Study the drawing (mm; zero at the part's minimum x, y, z) and answer. Coordinates: 2 decimals unless noted, no trailing zeros. Loops run counter-clockwise (first coordinate to the right, second up) from the corner with the lowest first, then second, coordinate; pieces in that order, holes last.
Q1. Straight lines are drawn through the part: line 1 (X direction, y = 62.5, z = 31) (1 decimal); line 2 (Y direction, x = 68, z = 68) (1 decimal); line 3 (Y direction, x = 60, z = 64) (1 decimal). For each, find the intervals that lie inside material, in ascending order.
Q2. Section A-A (z = 42) is taken. Give the vertices of the cut face in (x, y) (1 decimal).
Q3. The mould has two halves that part along X. Classify the marked faces 1 and 2: pulls with the +X half, pulls with the -X half, needs draft (parallel to the pull), parting line crosses it, or undercut.
Q4. Flat-ended cylindrical pins translate along their axes: P1, Ø12.5, axis at x = 59.56, y = 59.56, coming from the +Z side; P2, Ø5, axis at x = 53, z = 49.5, coming from the +Y side; P3, Ø5, axis at y = 49.5, z = 36, coming from the +X side (1 decimal); P4, Ø8, axis at x = 75, y = 78, coming from the -Z side. Find the tip coordinate at first contact, or state that the pin passes through.
Q5. Section B-B (z = 73) is taken. Give the vertices of the cut face in (x, y) (1 decimal).
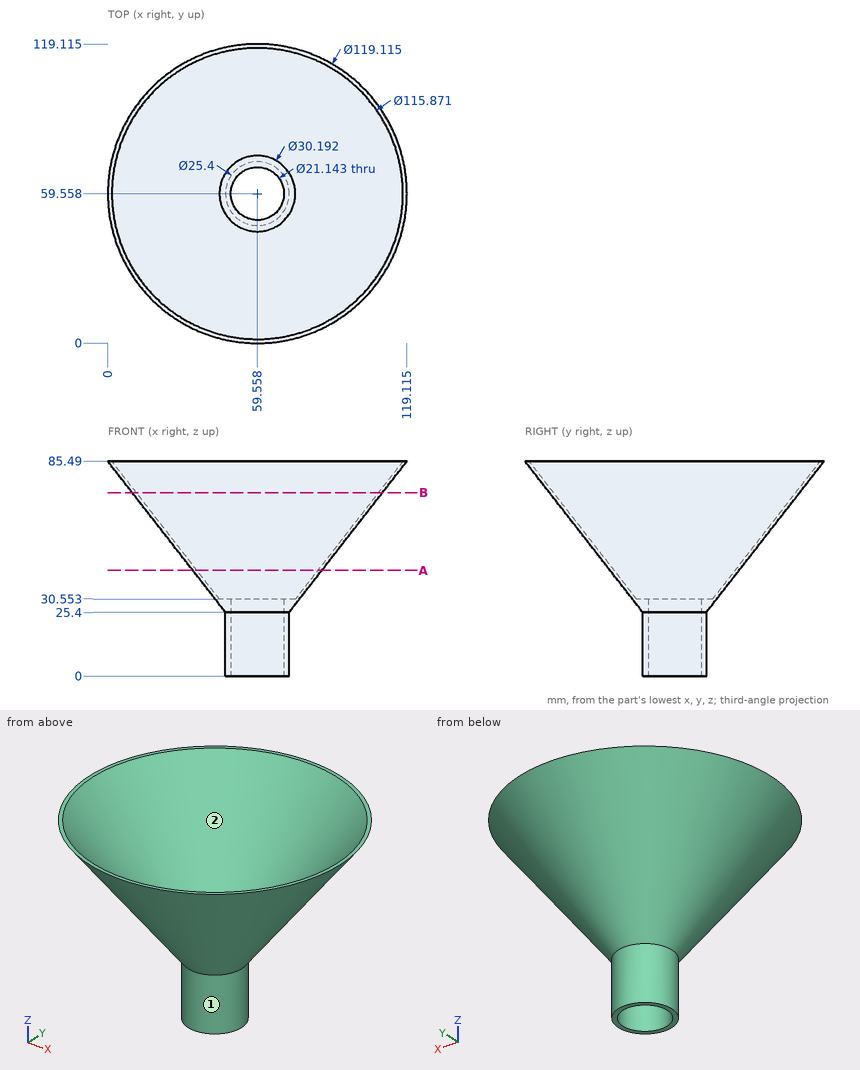
Numbers:
1. line 1: x = 42.7 to 44.4, 74.7 to 76.4
1. line 2: y = 14.4 to 16.1, 103 to 104.7
1. line 3: y = 16.8 to 18.4, 100.7 to 102.4
2. outline: circle Ø51.3 at (59.6, 59.6); hole circle Ø48 at (59.6, 59.6)
3. face 1: parting line crosses it
3. face 2: undercut
4. P1: passes through
4. P2: stops at y = 92.41
4. P3: stops at x = 80.4
4. P4: stops at z = 34.83
5. outline: circle Ø99.6 at (59.6, 59.6); hole circle Ø96.4 at (59.6, 59.6)
